from build123d import *

# Parameters (mm, degrees)
SKETCH1_W           = 86.36
SKETCH1_H           = 71.12
BOSS_EXTRUDE3_DEPTH = 50.8
SKETCH3_W           = 81.28
SKETCH3_H           = 66.04
CUT_EXTRUDE1_DEPTH  = 48.26
SKETCH4_R           = 1.524
BOSS_EXTRUDE7_DEPTH = 6.35


with BuildPart() as part:
    # Sketch1 → Boss-Extrude3 (new body)
    with BuildSketch(Plane(origin=(0, 0, 0), x_dir=(1, 0, 0), z_dir=(0, 1, 0))):
        with Locations((43.18, 35.56)):
            Rectangle(SKETCH1_W, SKETCH1_H)
    extrude(amount=BOSS_EXTRUDE3_DEPTH)

    # Sketch3 → Cut-Extrude1 (cut)
    with BuildSketch(Plane(origin=(0, 50.8, 0), x_dir=(1, 0, 0), z_dir=(0, 1, 0))):
        with Locations((43.18, 35.56)):
            Rectangle(SKETCH3_W, SKETCH3_H)
    extrude(amount=-CUT_EXTRUDE1_DEPTH, mode=Mode.SUBTRACT)

    # Sketch4 → Boss-Extrude7 (add)
    with BuildSketch(Plane(origin=(0, 2.54, 0), x_dir=(1, 0, 0), z_dir=(0, 1, 0))):
        with Locations(Location((27.94, 36.576, 0), (0, 0, 270))):
            Circle(SKETCH4_R)
        with Locations(Location((63.5, 36.576, 0), (0, 0, 270))):
            Circle(SKETCH4_R)
        with Locations(Location((63.5, 6.35, 0), (0, 0, 270))):
            Circle(SKETCH4_R)
        with Locations(Location((27.94, 6.35, 0), (0, 0, 270))):
            Circle(SKETCH4_R)
    extrude(amount=BOSS_EXTRUDE7_DEPTH)


solid = part.part
Verification items for the finished model (mm, model axes). A direction names the side the tool comes from. Give positions to 0.01 mm unless a question says otherwise; leave off trailing zeros. Loops run counter-clockwise (first coordinate to the right, second up) from the corner with the lowest first, then second, coordinate; pieces in that order, holes last. Notation, with made-up numbers: (6.25, -19.75) - (58.25, -19.75) arc R32 cw to (58.25, 14.25) - close; hole circle Ø2 at (-6.5, 49.25). An arc over 180 degrees is marked (long way). Write item = value, one per line. Start each with the question number.
Q1. Mould release check, pull along X, two halves, no side actions. Record for faces 1 (the face through (43, 25, -71.12)), 2 (the face through (0, 25, -35)), 3 (the face through (2.54, 27, -35)): released by +X, released by -X, zero draft, split by the parting line, or undercut.
Q2. Cross-section at A-A, the plane y = 16.5. Enter the section's corners in (x, z).
Q3. Cross-section at C-C, the plane z = -6.35. Enter the section's corners in (x, y).
Q4. Cross-section at B-B, the plane x = 41. Enter the section's corners in (y, z), and give its area (3 significant figures).
Q5. Cross-section at D-D, the plane x = 63.5. Enter the section's corners in (y, z).
Q6. Thickness scan on line 1 (X direction, y = 44, z = -13.5); line 2 (Z direction, x = 81.5, y = 42.5); line 3 (Y direction, x = 25, z = -11). Record the ranges inside material, lowest first.
Q7. Tool access check on faces 4 (the face through (40, 50.8, -1)), 5 (the face through (64, 8.89, -37)). Record the directions out of +Z, -Z, +X, -X, +Y, -Y that give a thin tool (end or side, any length) a straight path to the whole face; none if there is none.
Q8. Depth check by flat-ended pin: P1, Ø24, axis at x = 58, y = 33, coming from the +Z side; P2, Ø2, axis at x = 70, z = -34, coming from the +Y side; P3, Ø0.9, axis at x = 27, z = -5.5, coming from the +Y side. Enter the tip coordinate at first touch or a pass-through.
Answer key:
q1.face_1 = zero draft
q1.face_2 = released by -X
q1.face_3 = undercut
q2.outline = (0, -71.12) - (86.36, -71.12) - (86.36, 0) - (0, 0) - close; hole (2.54, -68.58) - (83.82, -68.58) - (83.82, -2.54) - (2.54, -2.54) - close
q3.outline = (0, 0) - (86.36, 0) - (86.36, 50.8) - (83.82, 50.8) - (83.82, 2.54) - (65.02, 2.54) - (65.02, 8.89) - (61.98, 8.89) - (61.98, 2.54) - (29.46, 2.54) - (29.46, 8.89) - (26.42, 8.89) - (26.42, 2.54) - (2.54, 2.54) - (2.54, 50.8) - (0, 50.8) - close
q4.outline = (0, -71.12) - (50.8, -71.12) - (50.8, -68.58) - (2.54, -68.58) - (2.54, -2.54) - (50.8, -2.54) - (50.8, 0) - (0, 0) - close
q4.area = 426 mm^2
q5.outline = (0, -71.12) - (50.8, -71.12) - (50.8, -68.58) - (2.54, -68.58) - (2.54, -38.1) - (8.89, -38.1) - (8.89, -35.05) - (2.54, -35.05) - (2.54, -7.87) - (8.89, -7.87) - (8.89, -4.83) - (2.54, -4.83) - (2.54, -2.54) - (50.8, -2.54) - (50.8, 0) - (0, 0) - close
q6.line_1 = 0 to 2.54, 83.82 to 86.36
q6.line_2 = -71.12 to -68.58, -2.54 to 0
q6.line_3 = 0 to 2.54
q7.face_4 = +Z, -Z, +X, -X, +Y
q7.face_5 = +Y
q8.P1 = 0
q8.P2 = 2.54
q8.P3 = 8.89
